Input: part model. Units: mm. Frame: model coordinates. Coordinates: 2 decimals unless noted, no trailing zeros. Loops run counter-clockwise (first coordinate to the right, second up) from the corner with the lowest first, then second, coordinate; pieces in that order, holes last. Notation, with made-up numbers: (69, 54.25) - (117, 54.25) arc R26 cw to (117, 79.25) - close; hole circle Ø4 at (-27.75, 15.25). An arc over 180 degrees is marked (long way). Use a Markdown table: item, result. Add a question column.
1. Contact query for flat-ended pins moving along their axis: P1, Ø2.5, axis at x = 0, z = 0, coming from the -Y side; P2, Ø1, axis at y = -2, z = 5, coming from the +X side; P3, Ø1, axis at y = -2.5, z = 5, coming from the -X side. Output: stop coordinate, or through.
2. Section query A-A on x = 0. Return the cut outline in (y, z) (3 decimals), then the cut area to 3 significant figures.
3. Section query B-B on z = 0. Return the cut outline in (x, y) (3 decimals).
4. Draft query along Z for faces 1 (the face through (1.1, 0, -2.4)), 2 (the face through (-5.158, -1.493, -3.955)), 3 (the face through (-1.13, -1.49, -0.87)). Return one class per face: released by +Z, released by -Z, zero draft, split by the parting line, or undercut.
5. Ray query, L1, parallel to Z at x = 0, y = -1.8 (3 decimals); L2, parallel to Z at x = 1, y = -1.9; L3, parallel to Z at x = 3, y = -1.8. Return the intervals inside material, ascending. Write a range as [from, to].
6. Section query C-C on y = -2.3. Return the cut outline in (x, z).
```python
from build123d import *

# Parameters (mm, degrees)
F0_R     = 6.5
F0_R_2   = 1.425
F1_DEPTH = 3
F2_R     = 1
F3_R     = 1
F4_R     = 1
F5_R     = 1


with BuildPart() as f1:
    # F0 (on Front) → F1 (new body)
    with BuildSketch(Plane.XZ):
        Circle(F0_R)
        Circle(F0_R_2, mode=Mode.SUBTRACT)
    extrude(amount=F1_DEPTH)

    # F2
    f2_edges = [f1.edges().sort_by_distance(p)[0] for p in [
        (-1.425, -3, 0),
    ]]
    fillet(f2_edges, radius=F2_R)

    # F3
    f3_edges = [f1.edges().sort_by_distance(p)[0] for p in [
        (-1.425, 0, 0),
    ]]
    fillet(f3_edges, radius=F3_R)

    # F4
    f4_edges = [f1.edges().sort_by_distance(p)[0] for p in [
        (-6.5, 0, 0),
    ]]
    fillet(f4_edges, radius=F4_R)

    # F5
    f5_edges = [f1.edges().sort_by_distance(p)[0] for p in [
        (-6.5, -3, 0),
    ]]
    fillet(f5_edges, radius=F5_R)


solid = f1.part
```
Resolved:
| question | item | result |
|---|---|---|
| 1 | P1 | through |
| 1 | P2 | x = 4.69 |
| 1 | P3 | x = -4.59 |
| 2 | outline | (-3, -5.5) arc R1 ccw to (-2, -6.5) - (-1, -6.5) arc R1 ccw to (0, -5.5) - (0, -2.425) arc R1 ccw to (-1, -1.425) - (-2, -1.425) arc R1 ccw to (-3, -2.425) - close; (-3, 2.425) arc R1 ccw to (-2, 1.425) - (-1, 1.425) arc R1 ccw to (0, 2.425) - (0, 5.5) arc R1 ccw to (-1, 6.5) - (-2, 6.5) arc R1 ccw to (-3, 5.5) - close |
| 2 | area | 28.7 mm² |
| 3 | outline | (-6.5, -2) arc R1 ccw to (-5.5, -3) - (-2.425, -3) arc R1 ccw to (-1.425, -2) - (-1.425, -1) arc R1 ccw to (-2.425, 0) - (-5.5, 0) arc R1 ccw to (-6.5, -1) - close; (1.425, -2) arc R1 ccw to (2.425, -3) - (5.5, -3) arc R1 ccw to (6.5, -2) - (6.5, -1) arc R1 ccw to (5.5, 0) - (2.425, 0) arc R1 ccw to (1.425, -1) - close |
| 4 | face 1 | zero draft |
| 4 | face 2 | split by the parting line |
| 4 | face 3 | undercut |
| 5 | L1 | [-6.5, -1.425], [1.425, 6.5] |
| 5 | L2 | [-6.42, -1.02], [1.02, 6.42] |
| 5 | L3 | [-5.77, 5.77] |
| 6 | outline | circle Ø12.91 at (0, 0); hole circle Ø2.94 at (0, 0) |
